For this review, take the finished solid that the model builds, in its own axes (mm). A direction names the side the tool comes from. Give positions to 0.01 mm unless a question says otherwise; leave off trailing zeros. Write each loop counter-clockwise with the first axis right and the second up, starting at its lowest first coordinate (ties: lowest second). Pieces come first, ordered by that corner, then holes. Notation, with made-up numbers: M 76.25,21 L 133.25,21 A19 ccw 133.25,39 Z; hole C 87,50.5 d5. An arc over 180 degrees is marked long. Write item = value, one per line.
```python
from build123d import *

# Parameters (mm, degrees)
F0_W      = 139.7
F0_H      = 38.1
F1_DEPTH  = 38.1
F2_R      = 31.75
F3_DEPTH  = 38.1
F4_W      = 119.38
F4_H      = 13.462
F5_DEPTH  = 38.101
F6_R      = 20.955
F7_DEPTH  = 38.101
F8_W      = 50.8
F8_H      = 38.1
F9_DEPTH  = 38.1
F10_R     = 12.7
F11_R     = 6.35
F12_R     = 1.27
F13_R     = 12.7
F14_R     = 6.731
F15_DEPTH = 38.101
F16_SIZE  = 2.54


with BuildPart() as f1:
    # F0 (on Top) → F1 (new body)
    with BuildSketch(Plane.XY):
        Rectangle(F0_W, F0_H)
    extrude(amount=F1_DEPTH)

    # F2 (on Top) → F3 (join, through all)
    with BuildSketch(Plane.XY):
        Circle(F2_R)
    extrude(amount=F3_DEPTH)

    # F4 (on Top) → F5 (cut, through all)
    with BuildSketch(Plane.XY):
        Rectangle(F4_W, F4_H)
    extrude(amount=F5_DEPTH, mode=Mode.SUBTRACT)

    # F6 (on Top) → F7 (cut, through all)
    with BuildSketch(Plane.XY):
        Circle(F6_R)
    extrude(amount=F7_DEPTH, mode=Mode.SUBTRACT)

    # F8 (on Top) → F9 (join, through all)
    with BuildSketch(Plane.XY):
        with Locations((-95.25, 0)):
            Rectangle(F8_W, F8_H)
    extrude(amount=F9_DEPTH)

    # F10
    f10_edges = [f1.edges().sort_by_distance(p)[0] for p in [
        (25.4, -19.05, 19.05),
        (-25.4, -19.05, 19.05),
        (25.4, 19.05, 19.05),
        (-25.4, 19.05, 19.05),
    ]]
    fillet(f10_edges, radius=F10_R)

    # F11
    f11_edges = [f1.edges().sort_by_distance(p)[0] for p in [
        (-19.844537, -6.731, 19.05),
        (19.844537, -6.731, 19.05),
        (19.844537, 6.731, 19.05),
        (-19.844537, 6.731, 19.05),
    ]]
    fillet(f11_edges, radius=F11_R)

    # F12
    f12_edges = [f1.edges().sort_by_distance(p)[0] for p in [
        (59.69, 6.731, 19.05),
        (-59.69, 6.731, 19.05),
        (-59.69, -6.731, 19.05),
        (59.69, -6.731, 19.05),
    ]]
    fillet(f12_edges, radius=F12_R)

    # F13
    f13_edges = [f1.edges().sort_by_distance(p)[0] for p in [
        (-58.42, 6.731, 19.05),
        (-58.42, -6.731, 19.05),
        (69.85, 19.05, 19.05),
        (69.85, -19.05, 19.05),
        (-120.65, -19.05, 19.05),
        (-120.65, 19.05, 19.05),
    ]]
    fillet(f13_edges, radius=F13_R)

    # F14 (on Top) → F15 (cut, through all)
    with BuildSketch(Plane.XY):
        with Locations((-101.5897616744, 0)):
            Circle(F14_R)
    extrude(amount=F15_DEPTH, mode=Mode.SUBTRACT)

    # F16
    f16_edges = [f1.edges().sort_by_distance(p)[0] for p in [
        (44.12926, 19.05, 38.1),
        (66.130256, 15.330256, 38.1),
        (26.308371, 19.992085, 38.1),
        (69.85, 0, 38.1),
        (0, 31.75, 38.1),
        (66.130256, -15.330256, 38.1),
        (-26.308371, 19.992085, 38.1),
        (44.12926, -19.05, 38.1),
        (-69.52926, 19.05, 38.1),
        (26.308371, -19.992085, 38.1),
        (-116.930256, 15.330256, 38.1),
        (0, -31.75, 38.1),
        (-120.65, 0, 38.1),
        (-26.308371, -19.992085, 38.1),
        (-116.930256, -15.330256, 38.1),
        (-69.52926, -19.05, 38.1),
        (-108.320762, 0, 38.1),
        (-41.193848, -6.731, 38.1),
        (-59.318026, -6.359026, 38.1),
        (-20.726924, -7.62024, 38.1),
        (-59.69, 0, 38.1),
        (0, -20.955, 38.1),
        (-59.318026, 6.359026, 38.1),
        (20.726924, -7.62024, 38.1),
        (-41.193848, 6.731, 38.1),
        (41.193848, -6.731, 38.1),
        (-20.726924, 7.62024, 38.1),
        (59.318026, -6.359026, 38.1),
        (0, 20.955, 38.1),
        (59.69, 0, 38.1),
        (20.726924, 7.62024, 38.1),
        (59.318026, 6.359026, 38.1),
        (41.193848, 6.731, 38.1),
        (44.12926, 19.05, 0),
        (66.130256, 15.330256, 0),
        (26.308371, 19.992085, 0),
        (69.85, 0, 0),
        (0, 31.75, 0),
        (66.130256, -15.330256, 0),
        (-26.308371, 19.992085, 0),
        (44.12926, -19.05, 0),
        (-69.52926, 19.05, 0),
        (26.308371, -19.992085, 0),
        (-116.930256, 15.330256, 0),
        (0, -31.75, 0),
        (-120.65, 0, 0),
        (-26.308371, -19.992085, 0),
        (-116.930256, -15.330256, 0),
        (-69.52926, -19.05, 0),
        (-108.320762, 0, 0),
        (41.193848, 6.731, 0),
        (59.318026, 6.359026, 0),
        (20.726924, 7.62024, 0),
        (59.69, 0, 0),
        (0, 20.955, 0),
        (59.318026, -6.359026, 0),
        (-20.726924, 7.62024, 0),
        (41.193848, -6.731, 0),
        (-41.193848, 6.731, 0),
        (20.726924, -7.62024, 0),
        (-59.318026, 6.359026, 0),
        (0, -20.955, 0),
        (-59.69, 0, 0),
        (-20.726924, -7.62024, 0),
        (-59.318026, -6.359026, 0),
        (-41.193848, -6.731, 0),
    ]]
    chamfer(f16_edges, length=F16_SIZE)


solid = f1.part
```
1. For line 1 along X through (y, z) = (0, 12); line 2 along Y through (x, z) = (-33.5, 32); line 3 along X through (y, z) = (-1, 24), list the stretches that pass through material, from the lowest coordinate up. Write a range as from..to.
Responses:
line_1 = -120.65..-108.32, -94.86..-59.69, 59.69..69.85
line_2 = -19.05..-6.73, 6.73..19.05
line_3 = -120.65..-108.25, -94.93..-59.69, 59.69..69.85
2. We need section B-B, the plane z = 15.5. Count the separate pieces of the cut face and the enclosed holes in it, then the cut area to 3 significant figures.
Responses:
separate_pieces = 1
enclosed_holes = 2
area = 5,450 mm2
3. Insertion check: P1, Ø16.5, axis at x = -52.5, z = 23, coming from the +Y side; P2, Ø8, axis at x = 40, z = 12.5, coming from the -Y side; P3, Ø12, axis at y = 19, z = 26, coming from the -X side. Each pin has a flat end and moves straight along its axis. Give the tip position at first contact, or say it passes through.
Responses:
P1 = 19.05
P2 = -19.05
P3 = -118.77
4. Machinability: for faces 4 (the face through (-0.314, -20.953, 18.819)), 5 (the face through (64.93, -13.961, 37.377)), 6 (the face through (-116.83, -15.43, 19.28)), 7 (the face through (-60.223, 7.225, 36.812)), 8 (the face through (60.25, -7.25, 1.25)), which of the approach directions +Z, -Z, +X, -X, +Y, -Y give a long, thin tool a straight path to every point of the face, cutting with its end or side? Answer none if there is none.
Responses:
face_4 = +Z, -Z
face_5 = +Z, +X, -Y
face_6 = +Z, -Z, -X, -Y
face_7 = +Z
face_8 = -Z
5. The part is to be moulded in two halves that separate along Y. For faces 1 (the face through (64.9, -13.94, 0.69)), 2 (the face through (60.223, -7.225, 36.812)), 3 (the face through (64.74, 14.1, 0.69)), say which applies: +Y half, -Y half, draft (parallel to the pull), parting line (faces both ways), or undercut.
Responses:
face_1 = -Y half
face_2 = undercut
face_3 = +Y half
6. We need section C-C, the plane x = -82. Write out the cut boundary in (y, z), then the cut area to 3 significant figures.
Responses:
outline = M -19.05,2.54 L -16.51,0 L 16.51,0 L 19.05,2.54 L 19.05,35.56 L 16.51,38.1 L -16.51,38.1 L -19.05,35.56 Z
area = 1,440 mm2
7. We need section A-A, the plane y = 0. Write out the cut boundary in (x, z).
Responses:
outline = M -120.65,2.54 L -118.11,0 L -110.86,0 L -108.32,2.54 L -108.32,35.56 L -110.86,38.1 L -118.11,38.1 L -120.65,35.56 Z; M -94.86,2.54 L -92.32,0 L -62.23,0 L -59.69,2.54 L -59.69,35.56 L -62.23,38.1 L -92.32,38.1 L -94.86,35.56 Z; M 59.69,2.54 L 62.23,0 L 67.31,0 L 69.85,2.54 L 69.85,35.56 L 67.31,38.1 L 62.23,38.1 L 59.69,35.56 Z
